Source: three-view drawing plus pictorial views. Frame: mm from the lowest corner of the part. A direction names the side the tool comes from. Give positions to 0.01 mm unless a question says otherwise; leave off trailing zeros. Loops run counter-clockwise (first coordinate to the right, second up) from the corner with the lowest first, then second, coordinate; pieces in that order, holes last. Notation, with made-up numbers: M -15.75,1.25 L -1.75,1.25 A26 cw -1.75,35.25 Z; hole C 51,-3.75 d10. An arc over 180 degrees is marked long. Answer as a JSON object with one key per item and string values. Group by question number.
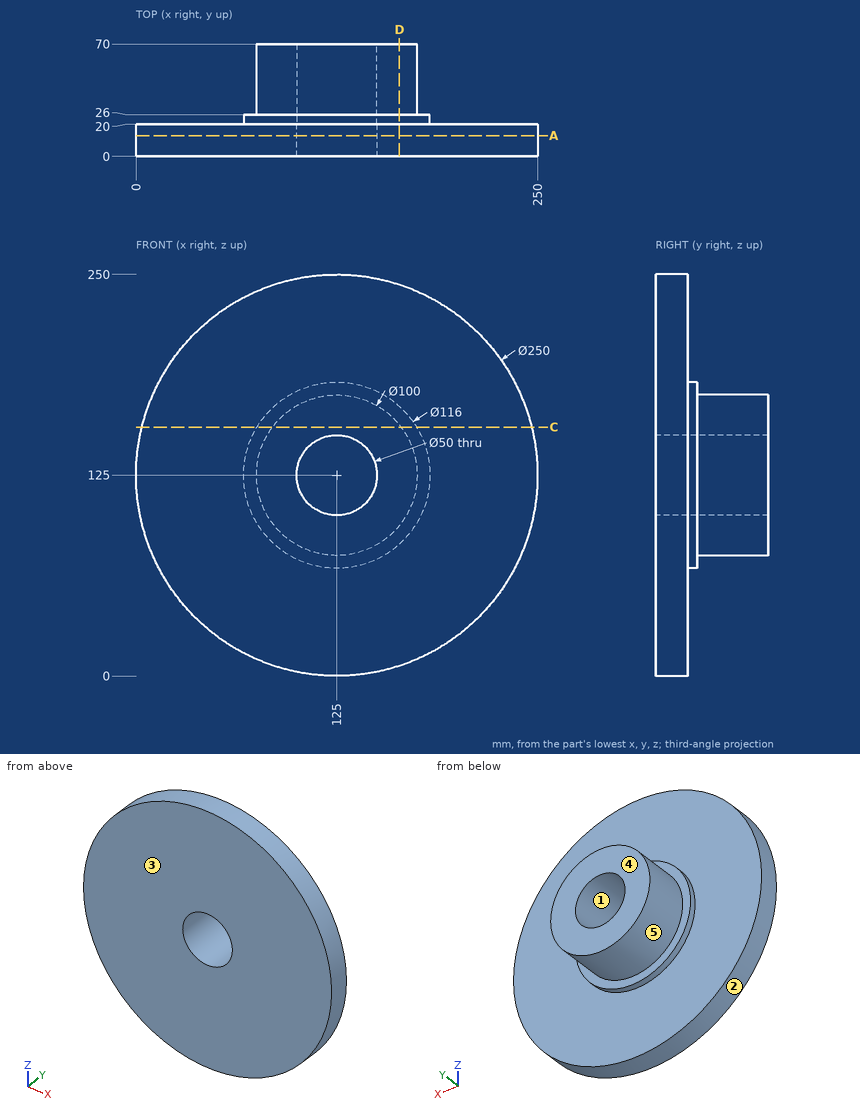
1. First-contact query: P1, Ø1, axis at x = 106, z = 63, coming from the +Y side; P2, Ø12, axis at y = 18.5, z = 96.5, coming from the +X side; P3, Ø4, axis at x = 55.5, y = 21.5, coming from the -Z side. Flat tips, straight axial feed; report the tip coordinate or a pass-through.
2. Section C-C (z = 155). Output: boundary loops of the cut face in (x, y).
3. Section D-D (x = 164). Output: boundary loops of the cut face in (y, z), then the cut area to 3 significant figures.
4. Section A-A (y = 13). Output: boundary loops of the cut face in (x, z).
5. Reachability of the marked faces 4 and 5 from +Z, -Z, +X, -X, +Y, -Y: full face, straight path, thin tool, end or side. Return the list, or none.
6. Material intervals for L1, parallel to X at y = 54.5, z = 125; L2, parallel to Z at x = 125, y = 17.5, sorted ascending.
7. Mould query, pull axis X, two halves, no side actions, for the marked faces 1, 2 and 3. Classes: pulls with the +X half, pulls with the -X half, needs draft (parallel to the pull), parting line crosses it, or undercut.
Geometry results:
{
 "1": {"P1": "y = 20", "P2": "x = 247.96", "P3": "z = 20.23"},
 "2": {"outline": "M 3.65,0 L 246.35,0 L 246.35,20 L 174.64,20 L 174.64,26 L 165,26 L 165,70 L 85,70 L 85,26 L 75.36,26 L 75.36,20 L 3.65,20 Z"},
 "3": {"outline": "M 0,6.24 L 20,6.24 L 20,82.07 L 26,82.07 L 26,93.71 L 70,93.71 L 70,156.29 L 26,156.29 L 26,167.93 L 20,167.93 L 20,243.76 L 0,243.76 Z", "area": "8,020 mm2"},
 "4": {"outline": "C 125,125 d250; hole C 125,125 d50"},
 "5": {"face 4": "+Z, -Z, +X, -X, +Y", "face 5": "+Y"},
 "6": {"L1": "75 to 100, 150 to 175", "L2": "0 to 100, 150 to 250"},
 "7": {"face 1": "undercut", "face 2": "parting line crosses it", "face 3": "needs draft"}
}
